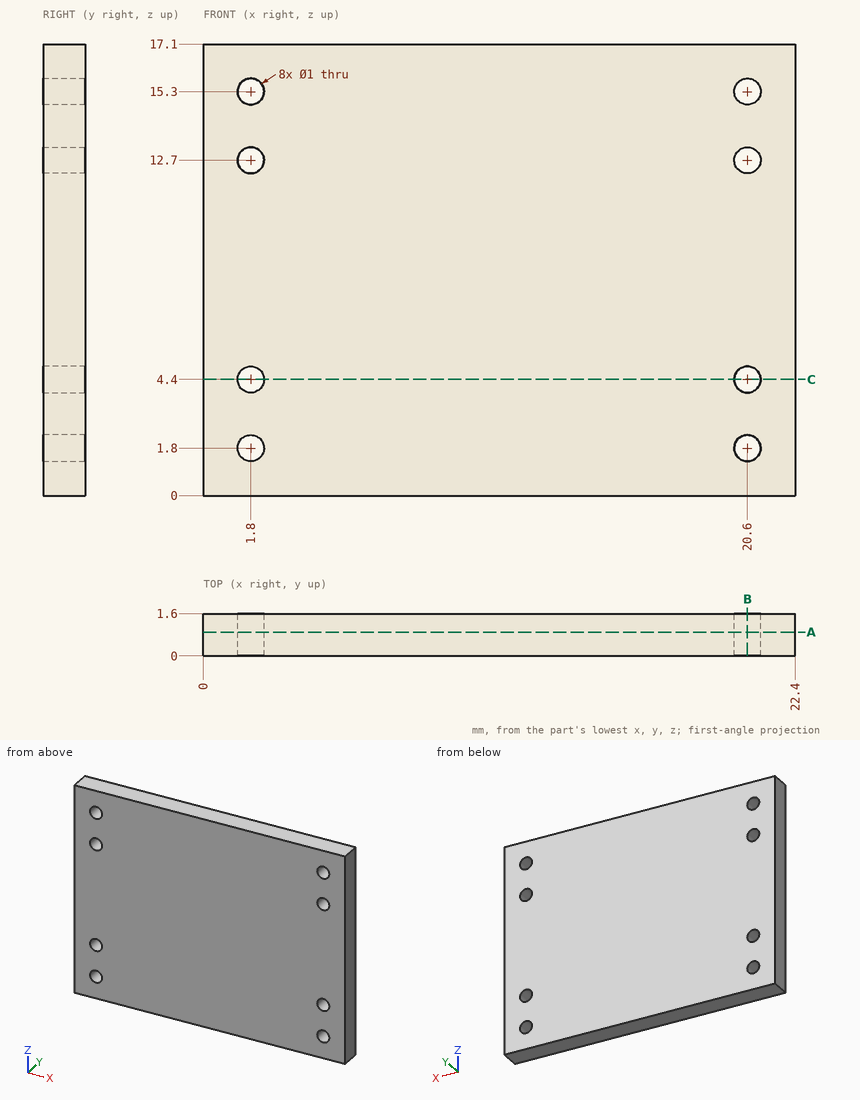
Answer from the drawing. Dimensions are ordinates in mm from the lowest x, y and z of the part. Round coordinates to 2 decimals unless told otherwise and drop trailing zeros. Loops run counter-clockwise (first coordinate to the right, second up) from the corner with the lowest first, then second, coordinate; pieces in that order, holes last. Notation, with made-up numbers: (13.5, 64) - (23.5, 64) arc R15 ccw to (23.5, 78) - close; hole circle Ø8 at (84, 10). An arc over 180 degrees is marked (long way). Return JSON: item names as keys, results as strings. Group by question number.
1. The part is cut by section A-A on y = 0.9. State how many separate pieces and enclosed holes the cut face has, then the cut area to 3 significant figures.
2. Consider probe 1 along Z at (x, y) = (20.6, 0.8); probe 2 along X at (y, z) = (0.3, 4.4). Determine where each line is inside the solid, lowest interval first.
3. The part is cut by section C-C on z = 4.4. Determine the outline of the cut face in (x, y).
4. The part is cut by section B-B on x = 20.6. Determine the outline of the cut face in (y, z), then the cut area to 3 significant figures.
Resolved:
{
 "1": {"separate pieces": "1", "enclosed holes": "8", "area": "377 mm²"},
 "2": {"probe 1": "z = 0 to 1.3, 2.3 to 3.9, 4.9 to 12.2, 13.2 to 14.8, 15.8 to 17.1", "probe 2": "x = 0 to 1.3, 2.3 to 20.1, 21.1 to 22.4"},
 "3": {"outline": "(0, 0) - (1.3, 0) - (1.3, 1.6) - (0, 1.6) - close; (2.3, 0) - (20.1, 0) - (20.1, 1.6) - (2.3, 1.6) - close; (21.1, 0) - (22.4, 0) - (22.4, 1.6) - (21.1, 1.6) - close"},
 "4": {"outline": "(0, 0) - (1.6, 0) - (1.6, 1.3) - (0, 1.3) - close; (0, 2.3) - (1.6, 2.3) - (1.6, 3.9) - (0, 3.9) - close; (0, 4.9) - (1.6, 4.9) - (1.6, 12.2) - (0, 12.2) - close; (0, 13.2) - (1.6, 13.2) - (1.6, 14.8) - (0, 14.8) - close; (0, 15.8) - (1.6, 15.8) - (1.6, 17.1) - (0, 17.1) - close", "area": "21.0 mm²"}
}
